Verification items for this drawing (mm, ordinates from the low corner). A direction names the side the tool comes from. Round coordinates to 2 decimals unless told otherwise and drop trailing zeros. Write each loop counter-clockwise with the first axis right and the second up, starting at its lowest first coordinate (ties: lowest second). Pieces come first, ordered by that corner, then holes. Notation, with made-up numbers: (47, -13.75) -> (99, -13.75) arc R21 ccw to (99, 12.25) -> close; hole circle Ø4 at (14, 67). An arc over 180 degrees is marked (long way). One line per item, written item: value.
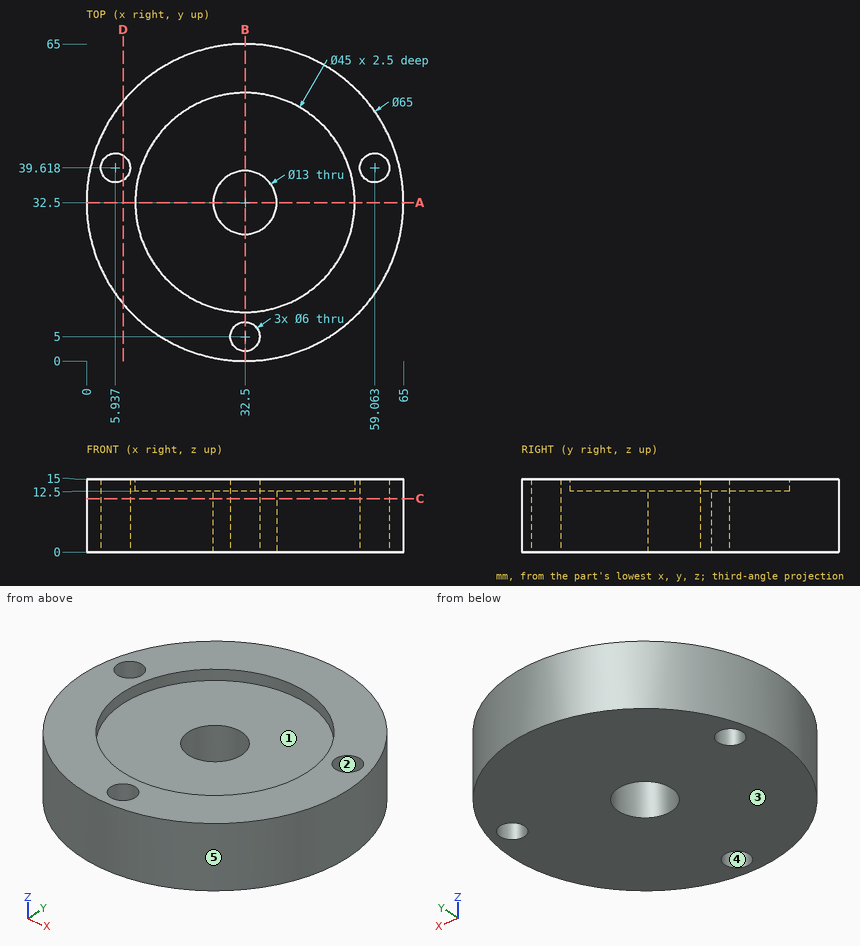
Item 1: Sectioned sample at C-C (z = 11). Enter the section's corners in (x, y).
Result set:
outline: circle Ø65 at (32.5, 32.5); hole circle Ø6 at (5.94, 39.62); hole circle Ø13 at (32.5, 32.5); hole circle Ø6 at (32.5, 5); hole circle Ø6 at (59.06, 39.62)
Item 2: Sectioned sample at A-A (y = 32.5). Enter the section's corners in (x, z), then the cut area to 3 significant figures.
Result set:
outline: (0, 0) -> (26, 0) -> (26, 12.5) -> (10, 12.5) -> (10, 15) -> (0, 15) -> close; (39, 0) -> (65, 0) -> (65, 15) -> (55, 15) -> (55, 12.5) -> (39, 12.5) -> close
area: 700 mm^2
Item 3: Release check for a two-part mould opening along Y. For the marked faces 3, 4 and 5 record: pulls with the +Y half, pulls with the -Y half, needs draft (parallel to the pull), parting line crosses it, or undercut.
Result set:
face 3: needs draft
face 4: undercut
face 5: parting line crosses it
Item 4: Depth check by flat-ended pin: pin 1 (3 mm diameter, centred on x = 19, y = 15.5, fed in from -Z); pin 2 (10.5 mm diameter, centred on x = 32.5, y = 32.5, fed in from +Z); pin 3 (22.5 mm diameter, centred on x = 25, y = 39.5, fed in from +Z); pin 4 (8 mm diameter, centred on y = 18, z = 6, fed in from -X). Enter the tip coordinate at first touch or a pass-through.
Result set:
pin 1: z = 0
pin 2: through
pin 3: z = 12.5
pin 4: x = 1.74
Item 5: Material ranges on line 1 along Y through (x, z) = (32.5, 13.25); line 2 along Y through (x, z) = (32.5, 4); line 3 along X through (y, z) = (41, 4.25) (1 decimal), recorded low to high.
Result set:
line 1: 0 to 2, 8 to 10, 55 to 65
line 2: 0 to 2, 8 to 26, 39 to 65
line 3: 1.1 to 3.3, 8.6 to 56.4, 61.7 to 63.9
Item 6: Sectioned sample at D-D (x = 7.5). Enter the section's corners in (y, z), then the cut area to 3 significant figures.
Result set:
outline: (11.73, 0) -> (37.06, 0) -> (37.06, 15) -> (11.73, 15) -> close; (42.18, 0) -> (53.27, 0) -> (53.27, 15) -> (42.18, 15) -> close
area: 546 mm^2
Item 7: Tool access check on the marked faces 1 and 2. Record the directions out of +Z, -Z, +X, -X, +Y, -Y that give a thin tool (end or side, any length) a straight path to the whole face; none if there is none.
Result set:
face 1: +Z
face 2: +Z, -Z
Item 8: Sectioned sample at B-B (x = 32.5). Enter the section's corners in (y, z), then the cut area to 3 significant figures.
Result set:
outline: (0, 0) -> (2, 0) -> (2, 15) -> (0, 15) -> close; (8, 0) -> (26, 0) -> (26, 12.5) -> (10, 12.5) -> (10, 15) -> (8, 15) -> close; (39, 0) -> (65, 0) -> (65, 15) -> (55, 15) -> (55, 12.5) -> (39, 12.5) -> close
area: 610 mm^2
